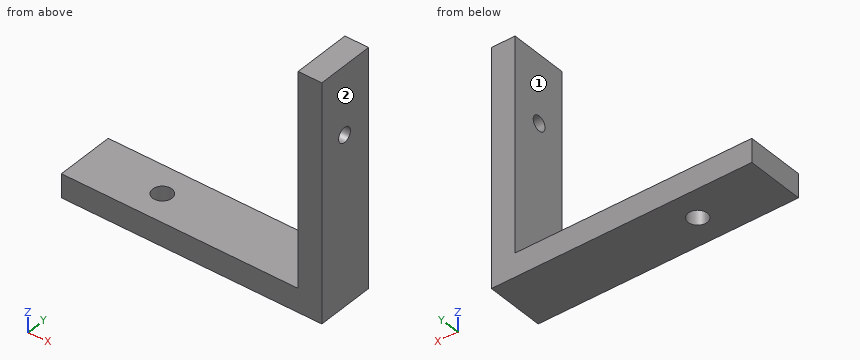
```python
from build123d import *

# Parameters (mm, degrees)
SKETCH_1_W      = 65.498017076
SKETCH_1_H      = 24.698375637
SKETCH_1_R      = 4.065381732
EXTRUDE_1_DEPTH = 10
SKETCH_2_W      = 34.501982924
SKETCH_2_H      = 24.698375637
EXTRUDE_2_DEPTH = 10
SKETCH_3_W      = 100
SKETCH_3_H      = 24.698375637
SKETCH_3_R      = 3.135440561
EXTRUDE_3_DEPTH = 10


with BuildPart() as part:
    # 草图1 → 凸台-拉伸1 (new body)
    with BuildSketch(Plane.XY):
        with Locations((39.890553187, 50.738604847)):
            Rectangle(SKETCH_1_W, SKETCH_1_H)
        with Locations((39.890553187, 50.738604847)):
            Circle(SKETCH_1_R, mode=Mode.SUBTRACT)
    extrude(amount=-EXTRUDE_1_DEPTH)

    # 草图2 → 凸台-拉伸2 (add)
    with BuildSketch(Plane(origin=(0, 0, -10), x_dir=(-1, 0, 0), z_dir=(0, 0, -1))):
        with Locations((-89.890553187, 50.738604847)):
            Rectangle(SKETCH_2_W, SKETCH_2_H)
    extrude(amount=-EXTRUDE_2_DEPTH)

    # 草图3 → 凸台-拉伸3 (add)
    with BuildSketch(Plane(origin=(107.141544649, 0, 0), x_dir=(0, 0, -1), z_dir=(1, 0, 0))):
        with Locations((-40, 50.738604847)):
            Rectangle(SKETCH_3_W, SKETCH_3_H)
        with Locations((-61.264027464, 50.387155503)):
            Circle(SKETCH_3_R, mode=Mode.SUBTRACT)
    extrude(amount=EXTRUDE_3_DEPTH)


solid = part.part
```
Geometry check sheet. Reference: the model listing, model coordinates, mm. Face numbers are marked on the shaded views. A direction names the side the tool comes from. Give positions to 0.01 mm unless a question says otherwise; leave off trailing zeros. Order: outer loops, then holes, each group sorted by start corner. A loop starts at its lowest first (then second) coordinate and runs counter-clockwise, first axis right, second up.
1. Section check C-C, the plane x = 57. Enter the section's corners in (y, z).
2. Thickness scan on L1, parallel to Z at x = 22, y = 47.25; L2, parallel to X at y = 40.5, z = 21; L3, parallel to X at y = 53.75, z = -5.5. Record the ranges inside material, lowest first.
3. Access from +Z, -Z, +X, -X, +Y, -Y to the whole of each face (thin tool, end or side, straight path). Record for the marked faces 1 and 2.
4. Section check A-A, the plane y = 52.25. Enter the section's corners in (x, z).
5. Section check D-D, the plane z = 80. Enter the section's corners in (x, y), and give its area (3 significant figures).
6. Section check B-B, the plane y = 57.75. Enter the section's corners in (x, z), and give its area (3 significant figures).
7. Gauge pin test, flat ends, axial feed: pin 1 Ø7.5 at (y, z) = (55.5, 34) entering from -X; pin 2 Ø7.5 at (x, y) = (64.5, 55.5) entering from +Z; pin 3 Ø6.5 at (x, y) = (39.89, 50.74) entering from +Z. Record the tip position at first contact, or that the pin passes through.
Values follow:
1. outline: (38.39, -10) - (63.09, -10) - (63.09, 0) - (38.39, 0) - close
2. L1: z = -10 to 0
2. L2: x = 107.14 to 117.14
2. L3: x = 7.14 to 37.16, 42.62 to 117.14
3. face 1: +Z, -X, +Y, -Y
3. face 2: +Z, -Z, +X, +Y, -Y
4. outline: (7.14, -10) - (36.12, -10) - (36.12, 0) - (7.14, 0) - close; (43.66, -10) - (117.14, -10) - (117.14, 58.74) - (107.14, 58.74) - (107.14, 0) - (43.66, 0) - close; (107.14, 63.79) - (117.14, 63.79) - (117.14, 90) - (107.14, 90) - close
5. outline: (107.14, 38.39) - (117.14, 38.39) - (117.14, 63.09) - (107.14, 63.09) - close
5. area: 247 mm2
6. outline: (7.14, -10) - (117.14, -10) - (117.14, 90) - (107.14, 90) - (107.14, 0) - (7.14, 0) - close
6. area: 2,000 mm2
7. pin 1: stops at x = 107.14
7. pin 2: stops at z = 0
7. pin 3: passes through
